Source: CAD feature listing. Evaluate the final solid. Frame: model axes, mm. Round coordinates to 2 decimals unless told otherwise and drop trailing zeros. Order: outer loops, then holes, each group sorted by start corner. A loop starts at its lowest first (then second) coordinate and runs counter-clockwise, first axis right, second up. Notation, with made-up numbers: (-11, 11) -> (47, 11) arc R12 ccw to (47, 25) -> close; hole circle Ø9 at (75, 17.5). An arc over 180 degrees is marked (long way). One line per item, written item: value. Start each with the question number.
1) Section B-B (x = -70). Return the cut outline in (y, z) (3 decimals), and give its area (3 significant figures).
2) Section C-C (z = -4.5). Return the cut outline in (x, y) (3 decimals).
3) Ray query, L1, parallel to Z at x = 0, y = 2; L2, parallel to Z at x = -55, y = 2.25; L3, parallel to Z at x = -0.5, y = 1.25. Return the intervals inside material, ascending.
4) Pin query (flat end, axial travel): P1, Ø1, axis at x = -37.5, y = 1.5, coming from the -Z side; P2, Ø1.5, axis at x = -20.5, y = 3, coming from the -Z side. Return the tip coordinate at first contact, or that it passes through.
5) Section A-A (y = 0.7). Return the cut outline in (x, z) (3 decimals).
6) Mould query, pull axis Z, two halves, no side actions, for faces 1 (the face through (2.374, 1.565, -0.748)), 2 (the face through (-7.543, 1.61, -0.695)), 3 (the face through (-24, 3.175, 3)). Classes: pulls with the +Z half, pulls with the -Z half, needs draft (parallel to the pull), parting line crosses it, or undercut.
```python
from build123d import *

# Parameters (mm, degrees)
SKETCH1_R           = 2.4892
BOSS_EXTRUDE1_DEPTH = 3.175
FILLET1_R           = 3.175
FILLET2_R           = 8.89


with BuildPart() as part:
    # Sketch1 → Boss-Extrude1 (new body)
    with BuildSketch(Plane(origin=(0, 0, 0), x_dir=(1, 0, 0), z_dir=(0, 1, 0))):
        with BuildLine():
            Line((-5.6642, 0), (-77.17919455, -4.935559597))
            Line((-77.17919455, -4.935559597), (-79.392042792, -6.182516957))
            Line((-79.392042792, -6.182516957), (-3.192042792, -6.978381463))
            Line((-3.192042792, -6.978381463), (0, -5.6642))
            ThreePointArc((0, -5.6642), (4.00519423, 4.00519423), (-5.6642, 0))
        make_face()
        Circle(SKETCH1_R, mode=Mode.SUBTRACT)
    extrude(amount=BOSS_EXTRUDE1_DEPTH)

    # Fillet1
    fillet1_edges = [part.edges().sort_by_distance(p)[0] for p in [
        (0, 1.5875, 5.6642),
        (-3.192042792, 1.5875, 6.978381463),
        (-77.17919455, 1.5875, 4.935559597),
    ]]
    fillet(fillet1_edges, radius=FILLET1_R)

    # Fillet2
    fillet2_edges = [part.edges().sort_by_distance(p)[0] for p in [
        (-5.6642, 1.5875, 0),
    ]]
    fillet(fillet2_edges, radius=FILLET2_R)


solid = part.part
```
Findings:
1. outline: (0, 4.44) -> (3.175, 4.44) -> (3.175, 6.281) -> (0, 6.281) -> close
1. area: 5.84 mm2
2. outline: (-3.44, 0) -> (3.44, 0) -> (3.44, 3.175) -> (-3.44, 3.175) -> close
3. L1: -5.66 to -2.49, 2.49 to 5.71
3. L2: 3.4 to 6.44
3. L3: -5.64 to -2.44, 2.44 to 5.87
4. P1: z = 2.16
4. P2: z = 0.97
5. outline: (-79.392, 6.183) -> (-77.804, 5.288) arc R3.175 ccw to (-76.464, 4.886) -> (-11.212, 0.383) arc R8.89 cw to (-4.602, -3.303) arc R5.664 ccw (long way) to (0.445, 5.647) arc R3.175 cw to (-0.514, 5.876) -> (-2.595, 6.733) arc R3.175 ccw to (-3.837, 6.972) -> close; hole circle Ø4.978 at (0, 0)
6. face 1: undercut
6. face 2: pulls with the -Z half
6. face 3: needs draft
